from build123d import *

# Parameters (mm, degrees)
SKETCH1_R           = 3.175
BOSS_EXTRUDE1_DEPTH = 12.7
SKETCH2_R           = 5.08
BOSS_EXTRUDE2_DEPTH = 0.127


with BuildPart() as part:
    # Sketch1 → Boss-Extrude1 (new body)
    with BuildSketch(Plane(origin=(0, 0, 0), x_dir=(1, 0, 0), z_dir=(0, 1, 0))):
        with Locations(Location((0, 0, 0), (0, 0, 270))):
            Circle(SKETCH1_R)
    extrude(amount=BOSS_EXTRUDE1_DEPTH)

    # Sketch2 → Boss-Extrude2 (add)
    with BuildSketch(Plane(origin=(0, 12.7, 0), x_dir=(1, 0, 0), z_dir=(0, 1, 0))):
        with Locations(Location((0, 0, 0), (0, 0, 270))):
            Circle(SKETCH2_R)
    extrude(amount=BOSS_EXTRUDE2_DEPTH)

    # Sketch3 → Revolve1 (revolve)
    with BuildSketch(Plane.XY):
        with BuildLine():
            Line((0, 12.827), (-3.886329239, 12.827))
            ThreePointArc((-3.886329239, 12.827), (-2.434866775, 14.914777268), (0, 15.647567139))
            Line((0, 15.647567139), (0, 12.827))
        make_face()
    revolve(axis=Axis((0, 12.827, 0), (0, 1, 0)))


solid = part.part
Geometry: final body of the model. Coordinates: model frame, mm. A direction names the side the tool comes from. Give positions to 0.01 mm unless a question says otherwise; leave off trailing zeros. Order: outer loops, then holes, each group sorted by start corner. A loop starts at its lowest first (then second) coordinate and runs counter-clockwise, first axis right, second up. Notation, with made-up numbers: (43, 87.5) -> (67, 87.5) arc R21 cw to (67, 113.5) -> close; hole circle Ø4 at (-1.75, 51.5). An arc over 180 degrees is marked (long way). Answer as a JSON object with one key per item and string values.
Q1. First-contact query: pin 1 (3 mm diameter, centred on x = 0, y = 6, fed in from +Z) (3 decimals); pin 2 (2 mm diameter, centred on x = 2.5, y = 13, fed in from -Z). Flat tips, straight axial feed; report the tip coordinate or a pass-through.
Entries:
{"pin 1": "stops at z = 3.175", "pin 2": "stops at z = -4.85"}
Q2. Access query for faces 1 (the flat face through (0, 0, 0)), 2 (the flat face through (-1.1, 12.7, 3.3)). Directions: +Z, -Z, +X, -X, +Y, -Y. A direction counts if a zero-diameter tool reaches every point of the face in a straight line with its end or side. Return the directions, or none.
Entries:
{"face 1": "+Z, -Z, +X, -X, -Y", "face 2": "-Y"}
Q3. Material intervals for probe 1 along Y at (x, z) = (-1.5, -0.75); probe 2 along X at (y, z) = (8.75, 1.75); probe 3 along Z at (x, y) = (2.5, 8), sorted ascending.
Entries:
{"probe 1": "y = 0 to 15.34", "probe 2": "x = -2.65 to 2.65", "probe 3": "z = -1.96 to 1.96"}
Q4. Section A-A (y = 9). Output: boundary loops of the cut face in (x, z) (3 decimals).
Entries:
{"outline": "circle Ø6.35 at (0, 0)"}
